Build history of the part. All positions in model axes, mm. Face numbers are marked on the shaded views. A direction names the side the tool comes from. Coordinates: 2 decimals unless noted, no trailing zeros. Write each loop counter-clockwise with the first axis right and the second up, starting at its lowest first coordinate (ties: lowest second). Pieces come first, ordered by that corner, then holes. Notation, with made-up numbers: M 23.25,65 L 71.25,65 A24 ccw 71.25,78 Z; hole C 74.25,56.5 d9. An arc over 180 degrees is marked long. Use CSV: the item, a comma, the result in double quotes. Start each with the question number.
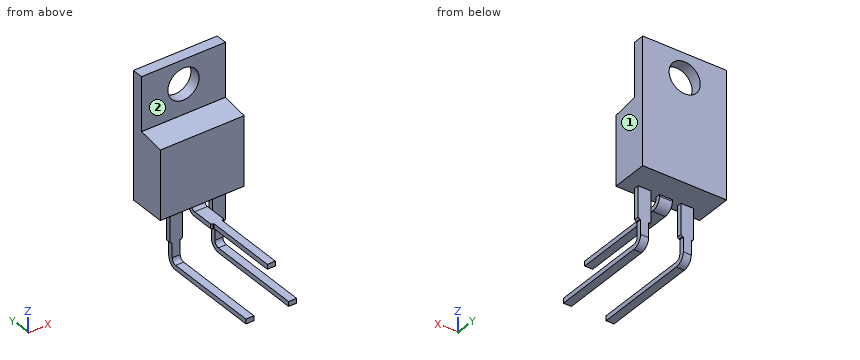
```python
from build123d import *

# Parameters (mm, degrees)
CORTAR_EXTRUIR1_START       = 1.8
CORTAR_EXTRUIR1_OUTLINE_W   = 10.5
CORTAR_EXTRUIR1_OUTLINE_H   = 15.8
CORTAR_EXTRUIR1_OUTLINE_R   = 1.95
CORTAR_EXTRUIR1_DEPTH       = 1.4
CORTAR_EXTRUIR1_START_2     = -0.6
CORTAR_EXTRUIR1_2_DEPTH     = 0.6
CORTAR_EXTRUIR1_START_3     = 1.79
CORTAR_EXTRUIR1_3_OUTLINE_W = 10.5
CORTAR_EXTRUIR1_3_OUTLINE_H = 9.1
CORTAR_EXTRUIR1_3_DEPTH     = 0.01
CORTAR_EXTRUIR1_START_4     = -5.25
CORTAR_EXTRUIR1_4_DEPTH     = 10.5
CROQUIS2_W                  = 1.6
CROQUIS2_H                  = 4.4
CORTAR_EXTRUIR2_DEPTH       = 10
EXTRUIR_L_MINA1_DEPTH       = 0.8
CROQUIS5_W                  = 8.6
CROQUIS5_H                  = 0.6
CORTAR_EXTRUIR3_DEPTH       = 25.279546948
EXTRUIR_L_MINA2_DEPTH       = 0.5
CUT_EXTRUDE1_DEPTH          = 10


with BuildPart() as part:
    # Cortar-Extruir1: read off the stored shape, not the designer's step
    # Cortar-Extruir1 outline → Cortar-Extruir1 (new body)
    with BuildSketch(Plane(origin=(0, -3.2, 0), x_dir=(1, 0, 0), z_dir=(0, 1, 0)).offset(CORTAR_EXTRUIR1_START)):
        with Locations((0, -7.9)):
            Rectangle(CORTAR_EXTRUIR1_OUTLINE_W, CORTAR_EXTRUIR1_OUTLINE_H)
        with Locations((0, -12.8)):
            Circle(CORTAR_EXTRUIR1_OUTLINE_R, mode=Mode.SUBTRACT)
    extrude(amount=CORTAR_EXTRUIR1_DEPTH)

    # Cortar-Extruir1 3 outline → Cortar-Extruir1 3 (add)
    with BuildSketch(Plane(origin=(0, -3.2, 0), x_dir=(1, 0, 0), z_dir=(0, 1, 0)).offset(CORTAR_EXTRUIR1_START_3)):
        with Locations((0, -4.55)):
            Rectangle(CORTAR_EXTRUIR1_3_OUTLINE_W, CORTAR_EXTRUIR1_3_OUTLINE_H)
    extrude(amount=CORTAR_EXTRUIR1_3_DEPTH)



with BuildPart() as body_2:
    # Cortar-Extruir1 2 outline → Cortar-Extruir1 2 (new body)
    with BuildSketch(Plane(origin=(0, -3.2, 0), x_dir=(1, 0, 0), z_dir=(0, 1, 0)).offset(CORTAR_EXTRUIR1_START_2)):
        Polygon((1.87, 0), (3.47, 0), (3.47, 3.8), (3.27, 4), (3.17, 4), (3.17, 14.4), (2.17, 14.4), (2.17, 4), (2.07, 4), (1.87, 3.8), align=None)
        Polygon((-0.8, 0), (0.8, 0), (0.8, 3.8), (0.6, 4), (0.5, 4), (0.5, 4.5), (-0.5, 4.5), (-0.5, 4), (-0.6, 4), (-0.8, 3.8), align=None)
        Polygon((-3.47, 0), (-1.87, 0), (-1.87, 3.8), (-2.07, 4), (-2.17, 4), (-2.17, 14.4), (-3.17, 14.4), (-3.17, 4), (-3.27, 4), (-3.47, 3.8), align=None)
    extrude(amount=CORTAR_EXTRUIR1_2_DEPTH)


with BuildPart() as part_1:
    add(part.part)

    add(body_2.part)  # Cortar-Extruir1 4 merges body 2
    # Cortar-Extruir1 4 outline → Cortar-Extruir1 4 (add)
    with BuildSketch(Plane.YZ.offset(CORTAR_EXTRUIR1_START_4)):
        Polygon((-1.41, 9.1), (-4.6, 8.6), (-4.6, 0), (-1.41, 0), align=None)
    extrude(amount=CORTAR_EXTRUIR1_4_DEPTH)

    # Croquis2 → Cortar-Extruir2 (cut)
    with BuildSketch(Plane(origin=(0, -3.2, 0), x_dir=(1, 0, 0), z_dir=(0, 1, 0))):
        with Locations((0, 2.3)):
            Rectangle(CROQUIS2_W, CROQUIS2_H)
    extrude(amount=-CORTAR_EXTRUIR2_DEPTH, mode=Mode.SUBTRACT)

    # Croquis3 → Extruir-Lámina1 (add, symmetric)
    with BuildSketch(Plane(origin=(0, 0, 0), x_dir=(0, 0, -1), z_dir=(1, 0, 0))):
        with BuildLine():
            Line((0.1, -3.8), (0.2, -3.8))
            ThreePointArc((0.2, -3.8), (0.624264069, -3.975735931), (0.8, -4.4))
            Line((0.8, -4.4), (0.8, -16.4))
            Line((0.8, -16.4), (1.4, -16.4))
            Line((1.4, -16.4), (1.4, -4.4))
            ThreePointArc((1.4, -4.4), (1.048528137, -3.551471863), (0.2, -3.2))
            Line((0.2, -3.2), (0.1, -3.2))
            Line((0.1, -3.2), (0.1, -3.8))
        make_face()
    extrude(amount=EXTRUIR_L_MINA1_DEPTH, both=True)

    # Croquis5 → Cortar-Extruir3 (cut, through all)
    with BuildSketch(Plane(origin=(3.17, 0, 0), x_dir=(0, 0, -1), z_dir=(1, 0, 0))):
        with Locations((10.1, -3.5)):
            Rectangle(CROQUIS5_W, CROQUIS5_H)
    extrude(amount=-CORTAR_EXTRUIR3_DEPTH, mode=Mode.SUBTRACT)

    # Croquis6 → Extruir-Lámina2 (add, symmetric)
    with BuildSketch(Plane(origin=(-2.67, 0, 0), x_dir=(0, 0, -1), z_dir=(1, 0, 0))):
        with BuildLine():
            ThreePointArc((5.8, -3.8), (6.224264069, -3.975735931), (6.4, -4.4))
            Line((6.4, -4.4), (6.4, -16.4))
            Line((6.4, -16.4), (7, -16.4))
            Line((7, -16.4), (7, -4.4))
            ThreePointArc((7, -4.4), (6.648528137, -3.551471863), (5.8, -3.2))
            Line((5.8, -3.2), (5.8, -3.8))
        make_face()
    extruir_l_mina2 = extrude(amount=EXTRUIR_L_MINA2_DEPTH, both=True)

    # Simetría1: Extruir-Lámina2 across plane
    add(extruir_l_mina2.mirror(Plane(origin=(0, 0, 0), x_dir=(0, 0, 1), z_dir=(1, 0, 0))))

    # Sketch2 → Cut-Extrude1 (cut)
    with BuildSketch(Plane(origin=(0, 0, -1.4), x_dir=(-1, 0, 0), z_dir=(0, 0, -1))):
        Polygon((-0.5, -16.4), (-0.5, -7.3), (-0.6, -7.3), (-0.8, -7.1), (-0.8, -16.4), align=None)
        Polygon((0.8, -16.4), (0.5, -16.4), (0.5, -7.3), (0.6, -7.3), (0.8, -7.1), align=None)
    extrude(amount=-CUT_EXTRUDE1_DEPTH, mode=Mode.SUBTRACT)


solid = part_1.part
```
1. Slice it at A-A (y = -9.75). List the corners of the cut face in (x, z), and give its area (3 significant figures).
2. Flat gauge pins, fed straight in: pin 1 (1.3 mm diameter, centred on x = -3, z = -2, fed in from -Y); pin 2 (1.5 mm diameter, centred on x = 3.5, y = -6, fed in from +Z); pin 3 (5 mm diameter, centred on x = -1, z = 13.5, fed in from -Y). Where does each tip first touch, or does it go through?
3. 3-axis set-ups, long thin cutter, end or side, ignore diameter. For the marked faces 1 and 2: which of +Z, -Z, +X, -X, +Y, -Y reach the whole face in a straight line?
4. Slice it at C-C (z = 12.8). List the corners of the cut face in (x, y), and give its area (3 significant figures).
5. Drill centre lines: line 1 along Z through (x, y) = (0, -0.75); line 2 along X through (y, z) = (-0.9, 12.8); line 3 along Y through (x, z) = (2.5, 1.25). Where is each one in solid material? Low to high. Write a range as from..to.
Established:
1,outline,"M -3.17,-7 L -2.17,-7 L -2.17,-6.4 L -3.17,-6.4 Z; M -0.5,-1.4 L 0.5,-1.4 L 0.5,-0.8 L -0.5,-0.8 Z; M 2.17,-7 L 3.17,-7 L 3.17,-6.4 L 2.17,-6.4 Z"
1,area,"1.80 mm2"
2,pin 1,"stops at y = -3.8"
2,pin 2,"stops at z = -6.4"
2,pin 3,"stops at y = -1.4"
3,face 1,"+Z, -Z, +X, +Y, -Y"
3,face 2,"+Z, +X, -X, -Y"
4,outline,"M -5.25,-1.4 L -1.95,-1.4 L -1.95,0 L -5.25,0 Z; M 1.95,-1.4 L 5.25,-1.4 L 5.25,0 L 1.95,0 Z"
4,area,"9.24 mm2"
5,line 1,"z = 0..10.85, 14.75..15.8"
5,line 2,"x = -5.25..-1.95, 1.95..5.25"
5,line 3,"y = -4.6..0"
